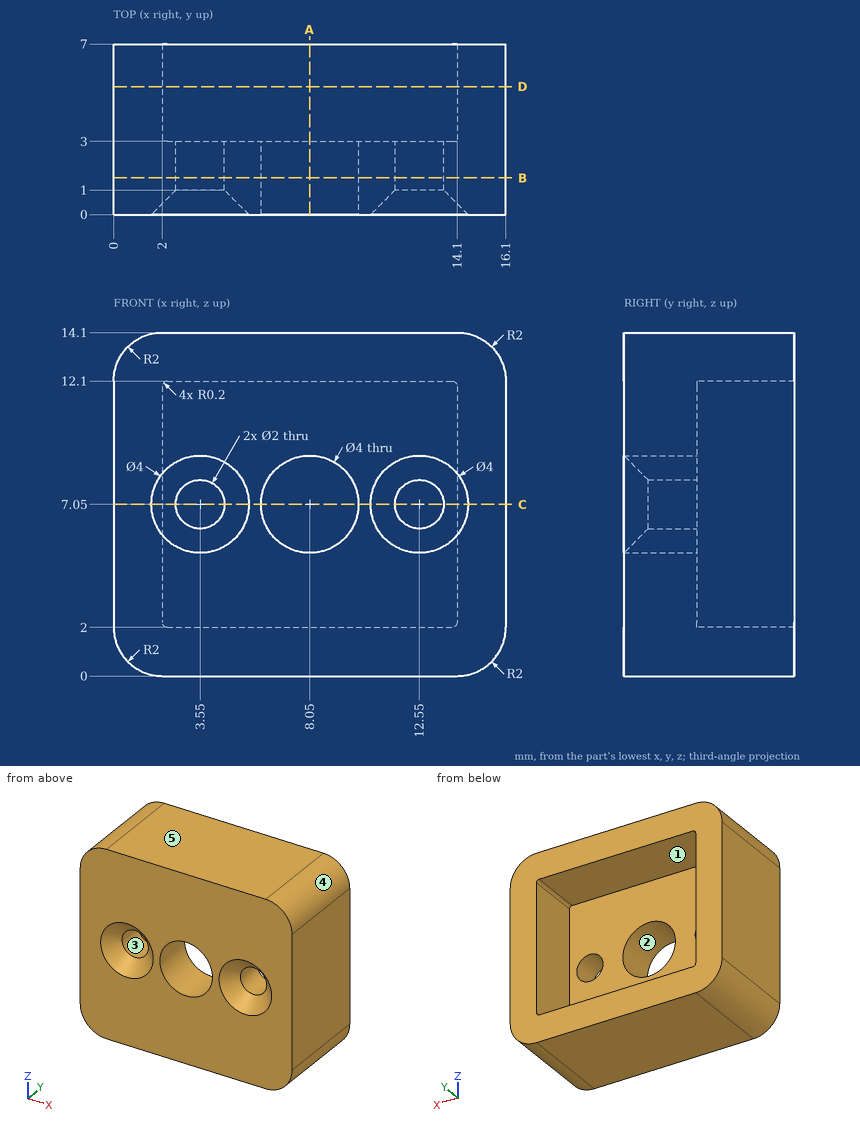
The figure shows three views and two pictorial views of one solid part (mm, origin at its lowest corner). Answer the questions. A direction names the side the tool comes from. Round coordinates to 2 decimals unless told otherwise and drop trailing zeros. Write each loop counter-clockwise with the first axis right and the second up, starting at its lowest first coordinate (ties: lowest second). Pieces come first, ordered by that corner, then holes. Notation, with made-up numbers: (-8.5, 31.5) - (34.5, 31.5) arc R31 ccw to (34.5, 62.5) - close; hole circle Ø7 at (-26.75, -21.75). An arc over 180 degrees is marked (long way). Use one line per item in the form item = value. Start each with the question number.
Item 1: A cutting plane is placed at D-D (y = 5.25). Write down the section's boundary in (x, z).
Item 2: A cutting plane is placed at C-C (z = 7.05). Write down the section's boundary in (x, y).
Item 3: Find the intervals of material crossed by line 1 (Z direction, x = 12.55, y = 1.7); line 2 (Z direction, x = 11.5, y = 5.25); line 3 (X direction, y = 4, z = 8.75), in increasing order. Write a range as [from, to].
Item 4: Determine the mould class of the marked faces 3, 4 and 5 for opening direction X: +X half, -X half, draft (parallel to the pull), parting line (faces both ways), or undercut.
Item 5: A tool of negligible diameter and unlimited length cuts with its end or side. For the marked faces 1 and 2, from which of +Z, -Z, +X, -X, +Y, -Y can it reach the whole face along a straight path? Write none if from no direction.
Item 6: Flat-ended cylindrical pins translate along their axes: pin 1 Ø2.5 at (x, z) = (12.55, 7.05) entering from -Y; pin 2 Ø3 at (x, z) = (7, 7.5) entering from +Y. Find the tip coordinate at first contact, or state that the pin passes through.
Item 7: A cutting plane is placed at A-A (x = 8.05). Write down the section's boundary in (y, z), plus the area to 3 significant figures.
Item 8: A cutting plane is placed at B-B (y = 1.5). Write down the section's boundary in (x, z), plus the area to 3 significant figures.
The answers:
q1.outline = (0, 2) arc R2 ccw to (2, 0) - (14.1, 0) arc R2 ccw to (16.1, 2) - (16.1, 12.1) arc R2 ccw to (14.1, 14.1) - (2, 14.1) arc R2 ccw to (0, 12.1) - close; hole (2, 2.2) arc R0.2 ccw to (2.2, 2) - (13.9, 2) arc R0.2 ccw to (14.1, 2.2) - (14.1, 11.9) arc R0.2 ccw to (13.9, 12.1) - (2.2, 12.1) arc R0.2 ccw to (2, 11.9) - close
q2.outline = (0, 0) - (1.55, 0) - (2.55, 1) - (2.55, 3) - (2, 3) - (2, 7) - (0, 7) - close; (4.55, 1) - (5.55, 0) - (6.05, 0) - (6.05, 3) - (4.55, 3) - close; (10.05, 0) - (10.55, 0) - (11.55, 1) - (11.55, 3) - (10.05, 3) - close; (13.55, 1) - (14.55, 0) - (16.1, 0) - (16.1, 7) - (14.1, 7) - (14.1, 3) - (13.55, 3) - close
q3.line_1 = [0, 6.05], [8.05, 14.1]
q3.line_2 = [0, 2], [12.1, 14.1]
q3.line_3 = [0, 2], [14.1, 16.1]
q4.face_3 = undercut
q4.face_4 = +X half
q4.face_5 = draft
q5.face_1 = +Y
q5.face_2 = +Y, -Y
q6.pin_1 = 0.75
q6.pin_2 = 3
q7.outline = (0, 0) - (7, 0) - (7, 2) - (3, 2) - (3, 5.05) - (0, 5.05) - close; (0, 9.05) - (3, 9.05) - (3, 12.1) - (7, 12.1) - (7, 14.1) - (0, 14.1) - close
q7.area = 46.3 mm^2
q8.outline = (0, 2) arc R2 ccw to (2, 0) - (14.1, 0) arc R2 ccw to (16.1, 2) - (16.1, 12.1) arc R2 ccw to (14.1, 14.1) - (2, 14.1) arc R2 ccw to (0, 12.1) - close; hole circle Ø2 at (3.55, 7.05); hole circle Ø4 at (8.05, 7.05); hole circle Ø2 at (12.55, 7.05)
q8.area = 205 mm^2
